Could you check a few things on this model? Use its own coordinates, in mm. A direction names the side the tool comes from. Coordinates: 2 decimals unless noted, no trailing zeros. Loops run counter-clockwise (first coordinate to the right, second up) from the corner with the lowest first, then second, coordinate; pieces in that order, holes last.
Autodesk Inventor part; units mm, degrees
ref_plane "YZ Plane" through (0, 0, 0) normal (1, 0, 0) x (0, 1, 0)
ref_plane "XZ Plane" through (0, 0, 0) normal (0, 1, 0) x (-1, 0, 0)
ref_plane "XY Plane" through (0, 0, 0) normal (0, 0, 1) x (1, 0, 0)
sketch "Sketch1" plane through (0, 0, 0) normal (0, 0, 1) x (1, 0, 0)
  line L0 (-152.4, -152.4) -> (152.4, -152.4)
  line L1 (152.4, -152.4) -> (152.4, 152.4)
  line L2 (152.4, 152.4) -> (-152.4, 152.4)
  line L3 (-152.4, 152.4) -> (-152.4, -152.4)
  line L4 (-152.4, -152.4) -> (152.4, 152.4) construction
  line L5 (152.4, -152.4) -> (-152.4, 152.4) construction
  point P0 (0, 0)
  dimension "d0" = 304.8
  dimension "d1" = 304.8
extrude "Extrusion1" add sketch "Sketch1" along normal blind 6.35
sketch "Sketch2" plane through (152.4, -152.4, 0) normal (1, 0, 0) x (0, 0, -1)
  line L0 (-6.35, 0) -> (-6.35, 304.8)
  line L1 (-6.35, 304.8) -> (-311.15, 304.8)
  line L2 (-311.15, 304.8) -> (-311.15, 0)
  line L3 (-311.15, 0) -> (-6.35, 0)
  line L4 (-6.35, 0) -> (-6.35, 304.8)
  line L5 (0, 0) -> (0, 304.8)
  line L6 (0, 304.8) -> (-6.35, 304.8)
  line L7 (-6.35, 0) -> (-6.35, 304.8)
  line L8 (0, 0) -> (-6.35, 0)
  point P0 (0, 152.4)
  dimension "d4" = 304.8
  dimension "d5" = 304.8
extrude "Extrusion2" add sketch "Sketch2" along normal blind 6.35
sketch "Sketch3" plane through (152.4, 152.4, 311.15) normal (0, 1, 0) x (1, 0, 0)
  line L0 (0, 304.8) -> (-304.8, 304.8)
  line L1 (0, 304.8) -> (0, 0)
  line L2 (0, 304.8) -> (-304.8, 304.8)
  line L3 (-304.8, 304.8) -> (-304.8, 0)
  line L4 (-304.8, 0) -> (0, 0)
  line L5 (0, 0) -> (0, 304.8)
  line L6 (-304.8, 311.15) -> (6.35, 311.15)
  line L7 (-304.8, 311.15) -> (-304.8, 304.8)
  line L8 (0, 304.8) -> (-304.8, 304.8)
  line L9 (0, 304.8) -> (0, 0)
  line L10 (0, 0) -> (6.35, 0)
  line L11 (6.35, 311.15) -> (6.35, 0)
  point P0 (-152.4, 311.15)
  dimension "d8" = 304.8
  dimension "d9" = 304.8
extrude "Extrusion3" add sketch "Sketch3" along normal blind 6.35
sketch "Sketch4" plane through (-152.4, 152.4, 6.35) normal (-1, 0, 0) x (0, 0, 1)
  line L0 (-6.35, -304.8) -> (-6.35, 6.35)
  line L1 (-6.35, -304.8) -> (0, -304.8)
  line L2 (0, 0) -> (0, -304.8)
  line L3 (0, 0) -> (304.8, 0)
  line L4 (304.8, 0) -> (304.8, 6.35)
  line L5 (-6.35, 6.35) -> (304.8, 6.35)
  line L6 (0, 0) -> (304.8, 0)
  line L7 (304.8, 0) -> (304.8, -304.8)
  line L8 (304.8, -304.8) -> (0, -304.8)
  line L9 (0, -304.8) -> (0, 0)
  point P0 (-6.35, -152.4)
  dimension "d12" = 304.8
  dimension "d13" = 304.8
extrude "Extrusion4" add sketch "Sketch4" along normal blind 6.35
sketch "Sketch5" plane through (152.4, -152.4, 6.35) normal (0, -1, 0) x (1, 0, 0)
  line L0 (6.35, -6.35) -> (-311.15, -6.35)
  line L1 (6.35, 304.8) -> (6.35, -6.35)
  line L2 (0, 304.8) -> (6.35, 304.8)
  line L3 (0, 304.8) -> (0, 0)
  line L4 (-304.8, 0) -> (0, 0)
  line L5 (-304.8, 0) -> (-304.8, 304.8)
  line L6 (-304.8, 304.8) -> (-311.15, 304.8)
  line L7 (-311.15, -6.35) -> (-311.15, 304.8)
  line L8 (-304.8, 0) -> (0, 0)
  line L9 (0, 0) -> (0, 304.8)
  line L10 (0, 304.8) -> (-304.8, 304.8)
  line L11 (-304.8, 304.8) -> (-304.8, 0)
  point P0 (-152.4, -6.35)
  dimension "d16" = 304.8
  dimension "d17" = 304.8
extrude "Extrusion5" add sketch "Sketch5" along normal blind 6.35
ref_plane "Work Plane1" through (152.4, 0, 311.15) normal (0, 1, 0) x (1, 0, 0)
ref_plane "Work Plane2" through (0, 152.4, 6.35) normal (-1, 0, 0) x (0, 0, 1)
properties part number "Robot Box" material "Wood (Birch)"
(1) For pin 1 (4 mm diameter, centred on x = -90.5, y = -3, fed in from -Z); pin 2 (4 mm diameter, centred on x = 75.5, y = 11.5, fed in from +Z), each with a flat end and sliding along its axis, tell me the tip position at first contact or that it passes through.
Answers:
pin 1: stops at z = 0
pin 2: stops at z = 6.35
(2) Imagine slicing it at B-B, the plane x = -137. Write out the boundary of the cut face in (y, z), and give its area (3 significant figures).
Answers:
outline: (-158.75, 0) - (158.75, 0) - (158.75, 311.15) - (152.4, 311.15) - (152.4, 6.35) - (-152.4, 6.35) - (-152.4, 311.15) - (-158.75, 311.15) - close
area: 5,890 mm2
(3) Which directions (+Z, -Z, +X, -X, +Y, -Y) give clear straight access to the entire face, cutting with the end or side of a thin tool? Please do faces 4 (the face through (-2, -158.75, 158)), 5 (the face through (-2, 152.4, 157)).
Answers:
face 4: +Z, -Z, +X, -X, -Y
face 5: +Z
(4) Imagine slicing it at A-A, the plane z = 281. Write out the boundary of the cut face in (x, y).
Answers:
outline: (-158.75, -158.75) - (158.75, -158.75) - (158.75, 158.75) - (-158.75, 158.75) - close; hole (-152.4, -152.4) - (152.4, -152.4) - (152.4, 152.4) - (-152.4, 152.4) - close
(5) I need wall thicknesses on probe 1 along X at (y, z) = (-93, 189); probe 2 along Z at (x, y) = (55, -111). Which ranges of each line are inside material? Lowest first, please.
Answers:
probe 1: x = -158.75 to -152.4, 152.4 to 158.75
probe 2: z = 0 to 6.35
(6) We'd pull the mould along Y, two halves only. Please class faces 1 (the face through (-2, 158.75, 153)), 2 (the face through (152.4, 2, 161)), 3 (the face through (-158.75, 2, 153)): +Y half, -Y half, draft (parallel to the pull), parting line (faces both ways), or undercut.
Answers:
face 1: +Y half
face 2: undercut
face 3: draft
